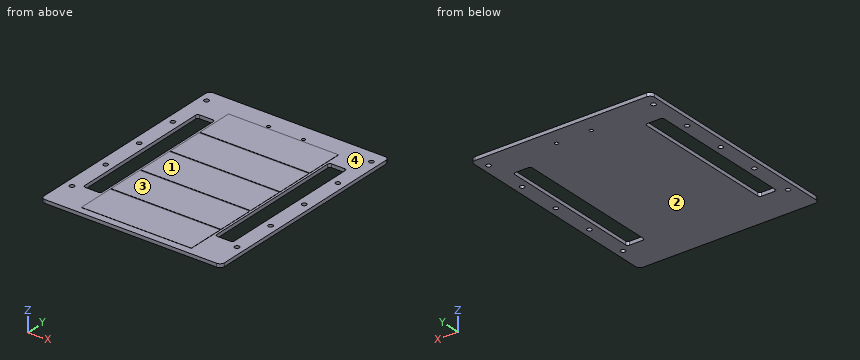
from build123d import *

# Parameters (mm, degrees)
SKETCH1_W          = 82
SKETCH1_H          = 100
BOARD_DEPTH        = 1.5875
SKETCH2_W          = 8
SKETCH2_H          = 68
ACCESS_HOLES_DEPTH = 65.680137262
SCREW_HOLES_D      = 2.1
CONNECTOR_HOLES_D  = 1.6
SKETCH4_W          = 50
SKETCH4_H          = 17.1
SOLAR_CELLS_DEPTH  = 0.1
OUTER_RADIUS_R     = 2
ACCESS_FILLET_R    = 1


with BuildPart() as part:
    # Sketch1 → board (new body)
    with BuildSketch(Plane.XY.offset(1.5875)):
        Rectangle(SKETCH1_W, SKETCH1_H)
    extrude(amount=-BOARD_DEPTH)

    # Sketch2 → access holes (cut, through all)
    with BuildSketch(Plane.XY.offset(1.5875)):
        with Locations((-30, 0)):
            Rectangle(SKETCH2_W, SKETCH2_H)
        with Locations((30, 0)):
            Rectangle(SKETCH2_W, SKETCH2_H)
    extrude(amount=-ACCESS_HOLES_DEPTH, mode=Mode.SUBTRACT)

    # screw holes (through all)
    with Locations(Plane(origin=(0, 0, 0), x_dir=(-1, 0, 0), z_dir=(0, 0, -1))):
        with Locations((37.5, 44), (37.5, 24), (37.5, 4), (37.5, -16), (37.5, -36), (-37.5, -36), (-37.5, -16), (-37.5, 4), (-37.5, 24), (-37.5, 44)):
            Hole(SCREW_HOLES_D / 2)

    # connector holes (through all)
    with Locations(Plane(origin=(0, 0, 0), x_dir=(-1, 0, 0), z_dir=(0, 0, -1))):
        with Locations((7.925, 42.25), (-7.925, 42.25)):
            Hole(CONNECTOR_HOLES_D / 2)

    # Sketch4 → solar cells (add)
    with BuildSketch(Plane.XY.offset(1.5875)):
        with Locations((0, 32.2)):
            Rectangle(SKETCH4_W, SKETCH4_H)
        with Locations((0, 14.6)):
            Rectangle(SKETCH4_W, SKETCH4_H)
        with Locations((0, -3)):
            Rectangle(SKETCH4_W, SKETCH4_H)
        with Locations((0, -20.6)):
            Rectangle(SKETCH4_W, SKETCH4_H)
        with Locations((0, -38.2)):
            Rectangle(SKETCH4_W, SKETCH4_H)
    extrude(amount=SOLAR_CELLS_DEPTH)

    # outer radius
    outer_radius_edges = [part.edges().sort_by_distance(p)[0] for p in [
        (-41, -50, 0.79375),
        (-41, 50, 0.79375),
        (41, 50, 0.79375),
        (41, -50, 0.79375),
    ]]
    fillet(outer_radius_edges, radius=OUTER_RADIUS_R)

    # access fillet
    access_fillet_edges = [part.edges().sort_by_distance(p)[0] for p in [
        (-26, 34, 0.79375),
        (-26, -34, 0.79375),
        (-34, -34, 0.79375),
        (-34, 34, 0.79375),
        (34, 34, 0.79375),
        (34, -34, 0.79375),
        (26, -34, 0.79375),
        (26, 34, 0.79375),
    ]]
    fillet(access_fillet_edges, radius=ACCESS_FILLET_R)


solid = part.part
Here's how the part is built. I have some questions about the finished solid (model axes, mm). Face numbers are marked on the shaded views. A direction names the side the tool comes from. Give positions to 0.01 mm unless a question says otherwise; leave off trailing zeros. Order: outer loops, then holes, each group sorted by start corner. A loop starts at its lowest first (then second) coordinate and runs counter-clockwise, first axis right, second up. Notation, with made-up numbers: M 78.25,46.25 L 130.25,46.25 A19 ccw 130.25,56.25 Z; hole C 63,20.5 d2. An arc over 180 degrees is marked long. Answer as a JSON object with one key per item and string values. Group by question number.
1) On a 3-axis mill with a long thin cutter (end or side, diameter ignored), from which of +Z, -Z, +X, -X, +Y, -Y can I reach the whole of each face in a straight line? I mean the marked faces 3 and 4. Say none if no direction works.
2) Suppose I cut it at B-B, the plane x = 37.5. Write out the boundary of the cut face in (y, z).
3) Suppose I cut it at A-A, the plane y = 4. Write out the boundary of the cut face in (x, z).
4) I'm going to push flat-ended pins straight in: pin 1 Ø2.5 at (x, y) = (37.5, -16) entering from -Z; pin 2 Ø2 at (x, y) = (-7.925, 42.25) entering from +Z. Where does each tip first touch, or does it pass through?
5) Please list where these lines run through material, in increasing order: L1, parallel to Y at x = -37.5, z = 0.45; L2, parallel to X at y = 30, z = 0.9; L3, parallel to Y at x = 37, z = 1.25. Write a range as [from, to].
6) Suppose I cut it at D-D, the plane z = 0.3. Count the separate pieces of the cut face and the enclosed holes in it, plus the area to 3 significant figures.
7) Suppose I cut it at C-C, the plane y = 39. Write out the boundary of the cut face in (x, z), plus the area to 3 significant figures.
8) We'd pull the mould along Z, two halves only. Please class the marked faces 1 and 2: pulls with the +Z half, pulls with the -Z half, needs draft (parallel to the pull), parting line crosses it, or undercut.
Results found:
{
 "1": {"face 3": "+Z, +X, -X, +Y, -Y", "face 4": "+Z"},
 "2": {"outline": "M -50,0 L -37.05,0 L -37.05,1.59 L -50,1.59 Z; M -34.95,0 L -17.05,0 L -17.05,1.59 L -34.95,1.59 Z; M -14.95,0 L 2.95,0 L 2.95,1.59 L -14.95,1.59 Z; M 5.05,0 L 22.95,0 L 22.95,1.59 L 5.05,1.59 Z; M 25.05,0 L 42.95,0 L 42.95,1.59 L 25.05,1.59 Z; M 45.05,0 L 50,0 L 50,1.59 L 45.05,1.59 Z"},
 "3": {"outline": "M -41,0 L -38.55,0 L -38.55,1.59 L -41,1.59 Z; M -36.45,0 L -34,0 L -34,1.59 L -36.45,1.59 Z; M -26,0 L 26,0 L 26,1.59 L 25,1.59 L 25,1.69 L -25,1.69 L -25,1.59 L -26,1.59 Z; M 34,0 L 36.45,0 L 36.45,1.59 L 34,1.59 Z; M 38.55,0 L 41,0 L 41,1.59 L 38.55,1.59 Z"},
 "4": {"pin 1": "z = 0", "pin 2": "z = 1.59"},
 "5": {"L1": "[-50, -37.05], [-34.95, -17.05], [-14.95, 2.95], [5.05, 22.95], [25.05, 42.95], [45.05, 50]", "L2": "[-41, -34], [-26, 26], [34, 41]", "L3": "[-50, -36.92], [-35.08, -16.92], [-15.08, 3.08], [4.92, 23.08], [24.92, 43.08], [44.92, 50]"},
 "6": {"separate pieces": "1", "enclosed holes": "14", "area": "7,070 mm²"},
 "7": {"outline": "M -41,0 L 41,0 L 41,1.59 L 25,1.59 L 25,1.69 L -25,1.69 L -25,1.59 L -41,1.59 Z", "area": "135 mm²"},
 "8": {"face 1": "pulls with the +Z half", "face 2": "pulls with the -Z half"}
}
